Verification items for the finished model (mm, model axes). A direction names the side the tool comes from. Round coordinates to 2 decimals unless told otherwise and drop trailing zeros. Order: outer loops, then holes, each group sorted by start corner. A loop starts at its lowest first (then second) coordinate and runs counter-clockwise, first axis right, second up. Notation, with made-up numbers: (82, 9.5) -> (109, 9.5) arc R14 cw to (109, 35.5) -> close; hole circle Ø2 at (80, -27.5). An arc over 180 degrees is marked (long way). Write item = value, one per line. Start each with the question number.
from build123d import *

# Parameters (mm, degrees)
BOSS_EXTRUDE3_DEPTH = 3.5
SKETCH6_W           = 4.5
SKETCH6_H           = 13.35
BOSS_EXTRUDE4_DEPTH = 2
SKETCH7_R           = 1.75
CUT_EXTRUDE2_DEPTH  = 16.123574313
BOSS_EXTRUDE7_DEPTH = 4.5
FILLET1_R           = 2


with BuildPart() as part:
    # Sketch5 → Boss-Extrude3 (new, symmetric)
    with BuildSketch(Plane.XY):
        Polygon((0, 0), (4.5, 0), (4.5, -13.35), (0, -13.35), (0, -11.35), (2.5, -11.35), (2.5, -8.175), (0, -8.175), (0, -5.175), (2.5, -5.175), (2.5, -2), (0, -2), align=None)
    extrude(amount=BOSS_EXTRUDE3_DEPTH, both=True)

    # Sketch6 → Boss-Extrude4 (add)
    with BuildSketch(Plane(origin=(0, 0, -3.5), x_dir=(-1, 0, 0), z_dir=(0, 0, -1))):
        with Locations((-2.25, -6.675)):
            Rectangle(SKETCH6_W, SKETCH6_H)
    extrude(amount=BOSS_EXTRUDE4_DEPTH)

    # Sketch7 → Cut-Extrude2 (cut, through all)
    with BuildSketch(Plane(origin=(0, 0, 0), x_dir=(1, 0, 0), z_dir=(0, 1, 0))):
        Circle(SKETCH7_R)
    extrude(amount=-CUT_EXTRUDE2_DEPTH, mode=Mode.SUBTRACT)

    # Sketch9 → Boss-Extrude7 (add, through all)
    with BuildSketch(Plane.ZY):
        with BuildLine():
            Line((-7.5, 3.175), (-5.5, 3.175))
            Line((-5.5, 3.175), (-5.5, 0))
            Line((-5.5, 0), (-5.5, -2))
            ThreePointArc((-5.5, -2), (-6.914213562, -1.414213562), (-7.5, 0))
            Line((-7.5, 0), (-7.5, 3.175))
        make_face()
    extrude(amount=-BOSS_EXTRUDE7_DEPTH)

    # Fillet1
    fillet1_edges = [part.edges().sort_by_distance(p)[0] for p in [
        (2.25, -2, -5.5),
    ]]
    fillet(fillet1_edges, radius=FILLET1_R)


solid = part.part
(1) Cross-section at A-A (z = -3.25). Enter the section's corners in (x, y) (3 decimals).
(2) Set-up check for faces 1 (the cylindrical face through (1.75, -6.65, 0.04)), 2 (the flat face through (2, 2, -5.5)), 3 (the flat face through (1, -10, -3.5)): record each of +Z, -Z, +X, -X, +Y, -Y from which the full face is reachable in a straight line by a thin tool's end or side.
(3) Draft check along Y on faces 4 (the flat face through (2.5, -4, 0)), 5 (the flat face through (2, 3.175, -7)), 6 (the cylindrical face through (1.75, -12.34, 0.04)). Enter one of: +Y half, -Y half, draft (parallel to the pull), parting line (faces both ways), or undercut.
(4) Cross-section at B-B (x = 3.45). Enter the section's corners in (y, z) (3 decimals), and give its area (3 significant figures).
(5) Cross-section at C-C (y = -12). Enter the section's corners in (x, z).
(6) Scan lines: line 1 along Y through (x, z) = (2.2, 2.75) (3 decimals); line 2 along X through (y, z) = (-1.75, 0); line 3 along Y through (x, z) = (3.7, -3.5). Record each from-to range of solid material in increasing order. Write a range as from..to.
(7) Cross-section at D-D (x = 0.75). Give the number of separate pieces and of enclosed holes in the cut face, and give its area (3 significant figures).
(8) Depth check by flat-ended pin: pin 1 (1.6 mm diameter, centred on x = 2, y = 2, fed in from +Z); pin 2 (0.8 mm diameter, centred on x = 2, z = 0.5, fed in from +Y); pin 3 (2.5 mm diameter, centred on y = -3.5, z = -0.5, fed in from -X). Enter the tip coordinate at first touch or a pass-through.
Outcome:
q1.outline = (0, -13.35) -> (4.5, -13.35) -> (4.5, 0) -> (0, 0) -> (0, -2) -> (2.5, -2) -> (2.5, -5.175) -> (0, -5.175) -> (0, -8.175) -> (2.5, -8.175) -> (2.5, -11.35) -> (0, -11.35) -> close
q2.face_1 = -X, +Y, -Y
q2.face_2 = +Z, +X, -X, +Y
q2.face_3 = +Z, -X
q3.face_4 = undercut
q3.face_5 = +Y half
q3.face_6 = draft
q4.outline = (-13.35, -5.5) -> (-3.464, -5.5) arc R2 cw to (-1.732, -6.5) arc R2 ccw to (0, -7.5) -> (3.175, -7.5) -> (3.175, -5.5) -> (0, -5.5) -> (0, 3.5) -> (-13.35, 3.5) -> close
q4.area = 130 mm^2
q5.outline = (0, -5.5) -> (4.5, -5.5) -> (4.5, 3.5) -> (0, 3.5) -> (0, 1.75) arc R1.75 cw to (0, -1.75) -> close
q6.line_1 = -13.35..-11.35, -8.175..-5.175, -2..0
q6.line_2 = 1.75..4.5
q6.line_3 = -13.35..0
q7.separate_pieces = 4
q7.enclosed_holes = 0
q7.area = 63.4 mm^2
q8.pin_1 = -5.5
q8.pin_2 = 0
q8.pin_3 = 2.5
